Model file for the job. Use its own axes, mm. Face numbers are marked on the shaded views. Round coordinates to 2 decimals unless told otherwise and drop trailing zeros. Order: outer loops, then holes, each group sorted by start corner. A loop starts at its lowest first (then second) coordinate and runs counter-clockwise, first axis right, second up. Notation, with made-up numbers: (3, 23) -> (54, 23) arc R35 cw to (54, 62) -> close; hole circle Ø7 at (64.5, 73.5). An arc over 180 degrees is marked (long way). Answer as CSV lines item,"result".
```python
from build123d import *

# Parameters (mm, degrees)
SKETCH_1_R      = 5.05
SKETCH_1_R_2    = 1.25
SKETCH_1_R_3    = 2.05
EXTRUDE_1_DEPTH = 2


with BuildPart() as part:
    # 草图1 → 凸台-拉伸1 (new body)
    with BuildSketch(Plane.XY):
        with BuildLine():
            Line((-15.488984032, 1), (-9.488984032, 1))
            ThreePointArc((-9.488984032, 1), (-4.998995168, 4.6), (-0.509006304, 1))
            Line((-0.509006304, 1), (5.001004832, 1))
            Line((5.001004832, 1), (39.492739898, 1))
            Line((39.492739898, 1), (39.492739898, 3.269234909))
            Line((39.492739898, 3.269234909), (5.001004832, 11.501004832))
            Line((5.001004832, 11.501004832), (3.407723631, 11.881256049))
            ThreePointArc((3.407723631, 11.881256049), (0.892865212, 10.016888454), (-0.509006304, 12.816019685))
            Line((-0.509006304, 12.816019685), (-38.998995168, 22.002009663))
            ThreePointArc((-38.998995168, 22.002009663), (-61.001004832, 0), (-38.998995168, -22.002009663))
            Line((-38.998995168, -22.002009663), (-0.509006304, -12.816019685))
            ThreePointArc((-0.509006304, -12.816019685), (0.892865212, -10.016888454), (3.407723631, -11.881256049))
            Line((3.407723631, -11.881256049), (5.001004832, -11.501004832))
            Line((5.001004832, -11.501004832), (5.001004832, -1))
            Line((5.001004832, -1), (-0.509006304, -1))
            ThreePointArc((-0.509006304, -1), (-4.998995168, -4.6), (-9.488984032, -1))
            Line((-9.488984032, -1), (-15.488984032, -1))
            Line((-15.488984032, -1), (-15.488984032, 1))
        make_face()
        with Locations((-38.998995168, 0)):
            Circle(SKETCH_1_R, mode=Mode.SUBTRACT)
        with Locations((-38.998995168, -11.5)):
            Circle(SKETCH_1_R_2, mode=Mode.SUBTRACT)
        with Locations((-12.498995168, -10)):
            Circle(SKETCH_1_R_3, mode=Mode.SUBTRACT)
        with Locations((-48.958287312, -5.75)):
            Circle(SKETCH_1_R_2, mode=Mode.SUBTRACT)
        with Locations(Location((-12.498995168, 10, 0), (0, 0, 180))):
            Circle(SKETCH_1_R_3, mode=Mode.SUBTRACT)
        with Locations((-48.958287312, 5.75)):
            Circle(SKETCH_1_R_2, mode=Mode.SUBTRACT)
        with Locations((-38.998995168, 11.5)):
            Circle(SKETCH_1_R_2, mode=Mode.SUBTRACT)
        with Locations((-29.039703025, 5.75)):
            Circle(SKETCH_1_R_2, mode=Mode.SUBTRACT)
        with Locations((-29.039703025, -5.75)):
            Circle(SKETCH_1_R_2, mode=Mode.SUBTRACT)
    extrude(amount=EXTRUDE_1_DEPTH)


solid = part.part
```
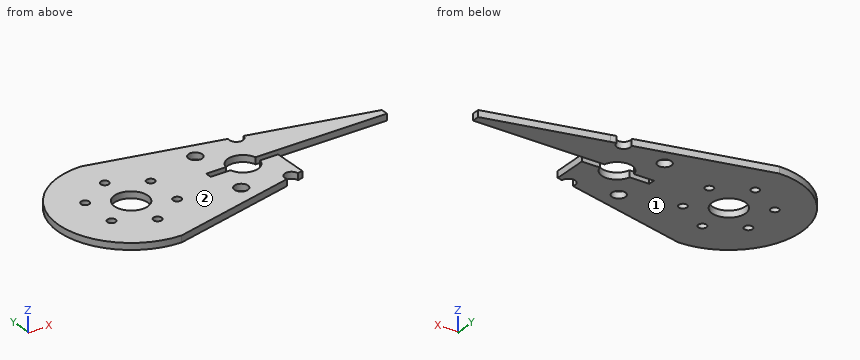
Q1. Flat gauge pins, fed straight in: pin 1 (2 mm diameter, centred on x = -48.96, y = -5.75, fed in from +Z); pin 2 (1 mm diameter, centred on x = -13.5, z = 1, fed in from -Y); pin 3 (1 mm diameter, centred on x = 12, z = 1, fed in from -Y); pin 4 (1 mm diameter, centred on y = -9, z = 0.5, fed in from +X). Where does each tip first touch, or does it go through?
Checks:
pin 1,"through"
pin 2,"y = -16.04"
pin 3,"y = 1"
pin 4,"x = 5"
Q2. Wall check: L1, parallel to Y at x = -39, z = 1; L2, parallel to Y at x = -28, z = 1.9; L3, parallel to X at y = -8.5, z = 0.7. Give the ranges that are in metal, low to high. Write a range as [from, to].
Checks:
L1,"[-22, -12.75], [-10.25, -5.05], [5.05, 10.25], [12.75, 22]"
L2,"[-19.38, -6.44], [-5.06, 5.06], [6.44, 19.38]"
L3,"[-59.29, -13.9], [-11.1, 5]"
Q3. Saw through at A-A (y = 0). Write the cut outline in (x, z), plus the area to 3 significant figures.
Checks:
outline,"(-61, 0) -> (-44.05, 0) -> (-44.05, 2) -> (-61, 2) -> close; (-33.95, 0) -> (-15.49, 0) -> (-15.49, 2) -> (-33.95, 2) -> close"
area,"70.8 mm²"
Q4. Mould opens along Z. For the marked faces 1 and 2 say: +Z half, -Z half, draft (parallel to the pull), parting line (faces both ways), or undercut.
Checks:
face 1,"-Z half"
face 2,"+Z half"
Q5. Saw through at B-B (z = 1.4). State how many separate pieces and enclosed holes the cut face has, plus the area to 3 significant figures.
Checks:
separate pieces,"1"
enclosed holes,"9"
area,"2,210 mm²"
Q6. Saw through at D-D (x = -18). Write the cut outline in (y, z).
Checks:
outline,"(-16.99, 0) -> (16.99, 0) -> (16.99, 2) -> (-16.99, 2) -> close"
Q7. Saw through at C-C (x = -3). Write the cut outline in (y, z), plus the area to 3 significant figures.
Checks:
outline,"(-13.41, 0) -> (-4.14, 0) -> (-4.14, 2) -> (-13.41, 2) -> close; (4.14, 0) -> (13.41, 0) -> (13.41, 2) -> (4.14, 2) -> close"
area,"37.1 mm²"
